```python
from build123d import *

# Parameters (mm, degrees)
SKETCH2_W            = 145.63575991
SKETCH2_H            = 16.06113598
BOSS_EXTRUDE1_DEPTH  = 80
SKETCH3_R            = 10
CUT_EXTRUDE1_DEPTH   = 110.363630747
BOSS_EXTRUDE2_DEPTH  = 20
SKETCH5_R            = 30
SKETCH5_R_2          = 10
BOSS_EXTRUDE3_DEPTH  = 100
FILLET1_R            = 5
BOSS_EXTRUDE9_REACH  = 183.085
BOSS_EXTRUDE10_DEPTH = 10
FILLET2_R            = 5
FILLET3_R            = 30


with BuildPart() as part:
    # Sketch2 → Boss-Extrude1 (new, symmetric)
    with BuildSketch(Plane(origin=(0, 0, 0), x_dir=(0, 0, -1), z_dir=(1, 0, 0))):
        Rectangle(SKETCH2_W, SKETCH2_H)
    extrude(amount=BOSS_EXTRUDE1_DEPTH, both=True)

    # Sketch3 → Cut-Extrude1 (cut, through all)
    with BuildSketch(Plane(origin=(0, 8.03056799, 0), x_dir=(1, 0, 0), z_dir=(0, 1, 0))):
        with Locations(Location((50, -42.817879955, 0), (0, 0, 270))):
            Circle(SKETCH3_R)
        with Locations(Location((-50, -42.817879955, 0), (0, 0, 270))):
            Circle(SKETCH3_R)
    extrude(amount=-CUT_EXTRUDE1_DEPTH, mode=Mode.SUBTRACT)

    # Sketch4 → Boss-Extrude2 (add)
    with BuildSketch(Plane(origin=(0, 0, -72.817879955), x_dir=(-1, 0, 0), z_dir=(0, 0, -1))):
        with BuildLine():
            Line((-26.680786367, 111.746822538), (-80, 8.03056799))
            Line((-80, 8.03056799), (80, 8.03056799))
            Line((80, 8.03056799), (26.680786367, 111.746822538))
            ThreePointArc((26.680786367, 111.746822538), (29.158391511, 105.086643705), (30, 98.03056799))
            ThreePointArc((30, 98.03056799), (-7.056075715, 68.872176479), (-26.680786367, 111.746822538))
        make_face()
    extrude(amount=-BOSS_EXTRUDE2_DEPTH)

    # Sketch5 → Boss-Extrude3 (add)
    with BuildSketch(Plane(origin=(0, 0, -72.817879955), x_dir=(-1, 0, 0), z_dir=(0, 0, -1))):
        with Locations((0, 98.03056799)):
            Circle(SKETCH5_R)
        with Locations((0, 98.03056799)):
            Circle(SKETCH5_R_2, mode=Mode.SUBTRACT)
    extrude(amount=-BOSS_EXTRUDE3_DEPTH)

    # Fillet1
    fillet1_edges = [part.edges().sort_by_distance(p)[0] for p in [
        (0, 8.03056799, -52.817879955),
    ]]
    fillet(fillet1_edges, radius=FILLET1_R)

    # Boss-Extrude9: up to this face of the body (flat: up to its plane)
    boss_extrude9_end = Plane(part.part.faces().sort_by_distance((0, 43.997298741, -52.817879955))[0])
    # Sketch12 → Boss-Extrude9 (add, up to the picked face)
    with BuildSketch(Plane.XY.offset(27.182120045), mode=Mode.PRIVATE) as boss_extrude9_sk1:
        with BuildLine():
            Line((10, 69.746296743), (10, 8.03056799))
            Line((10, 8.03056799), (-10, 8.03056799))
            Line((-10, 8.03056799), (-10, 69.746296743))
            ThreePointArc((-10, 69.746296743), (0, 68.03056799), (10, 69.746296743))
        make_face()
    boss_extrude9_tool1 = split(extrude(boss_extrude9_sk1.sketch, amount=-BOSS_EXTRUDE9_REACH, mode=Mode.PRIVATE), bisect_by=boss_extrude9_end, keep=Keep.BOTH, mode=Mode.PRIVATE)
    add(boss_extrude9_tool1.solids().sort_by(Axis((0, 38.315311, 27.18212), (0, 0, -1)))[0])

    # Sketch14 → Boss-Extrude10 (add, symmetric)
    with BuildSketch(Plane(origin=(0, 0, 0), x_dir=(0, 0, -1), z_dir=(1, 0, 0))):
        Polygon((-27.182120045, 69.746296743), (-72.817879955, 8.03056799), (-27.182120045, 8.03056799), align=None)
    extrude(amount=BOSS_EXTRUDE10_DEPTH, both=True)

    # Fillet2
    # the kernel refuses this fillet: 5 mm, written as the material it adds along each edge
    with BuildSketch(Plane(origin=(10, 13.03056799, -47.817879955), x_dir=(0, 0, -1), z_dir=(0, 1, 0))) as fillet2_piece_1:
        with BuildLine():
            CenterArc((5 - FILLET2_R, -FILLET2_R), FILLET2_R, 0, 90)
            Line((5, -FILLET2_R), (5, 0))
            Line((5, 0), (5 - FILLET2_R, 0))
        make_face()
    revolve(axis=Axis((10, 13.03056799, -47.817879955), (-1, 0, 0)), revolution_arc=90)
    with BuildSketch(Plane(origin=(-10, 13.03056799, -47.817879955), x_dir=(0, 0, -1), z_dir=(0, 1, 0))) as fillet2_piece_2:
        with BuildLine():
            CenterArc((5 - FILLET2_R, FILLET2_R), FILLET2_R, 270, 90)
            Line((5, FILLET2_R), (5, 0))
            Line((5, 0), (5 - FILLET2_R, 0))
        make_face()
    revolve(axis=Axis((-10, 13.03056799, -47.817879955), (-1, 0, 0)), revolution_arc=90)
    with BuildSketch(Plane(origin=(-10, 8.03056799, 72.817879955), x_dir=(-1, 0, 0), z_dir=(0, 0, -1))) as fillet2_piece_3_section:
        with BuildLine():
            CenterArc((FILLET2_R, FILLET2_R), FILLET2_R, 180, 90)
            Line((0, FILLET2_R), (0, 0))
            Line((0, 0), (FILLET2_R, 0))
        make_face()
    fillet2_piece_3 = extrude(amount=120.63575991, mode=Mode.PRIVATE)
    fillet2_piece_3 = split(fillet2_piece_3, bisect_by=Plane(origin=(-10, 8.03056799, 72.817879955), z_dir=(0, -0.5945577575874679, -0.8040529042871258)), keep=Keep.TOP, mode=Mode.PRIVATE)
    add(fillet2_piece_3)
    with BuildSketch(Plane(origin=(-10, 82.246296743, -52.817879955), x_dir=(0, 0, 1), z_dir=(0, -1, 0))) as fillet2_piece_4:
        with BuildLine():
            CenterArc((FILLET2_R, FILLET2_R), FILLET2_R, 180, 90)
            Line((0, FILLET2_R), (0, 0))
            Line((0, 0), (FILLET2_R, 0))
        make_face()
    extrude(amount=69.215728753)
    with BuildSketch(Plane(origin=(10, 13.03056799, -52.817879955), x_dir=(1, 0, 0), z_dir=(0, 1, 0))) as fillet2_piece_5:
        with BuildLine():
            CenterArc((FILLET2_R, -FILLET2_R), FILLET2_R, 90, 90)
            Line((0, -FILLET2_R), (0, 0))
            Line((0, 0), (FILLET2_R, 0))
        make_face()
    extrude(amount=69.215728753)
    with BuildSketch(Plane(origin=(10, 8.03056799, -47.817879955), x_dir=(1, 0, 0), z_dir=(0, 0, 1))) as fillet2_piece_6_section:
        with BuildLine():
            CenterArc((FILLET2_R, FILLET2_R), FILLET2_R, 180, 90)
            Line((0, FILLET2_R), (0, 0))
            Line((0, 0), (FILLET2_R, 0))
        make_face()
    fillet2_piece_6 = extrude(amount=120.63575991, mode=Mode.PRIVATE)
    fillet2_piece_6 = split(fillet2_piece_6, bisect_by=Plane(origin=(10, 65.701203771, 30.173268256), z_dir=(0, -0.5945577575874679, -0.8040529042871258)), keep=Keep.TOP, mode=Mode.PRIVATE)
    add(fillet2_piece_6)

    # Fillet3
    fillet3_edges = [part.edges().sort_by_distance(p)[0] for p in [
        (80, 0, 72.817879955),
        (-80, 0, 72.817879955),
    ]]
    fillet(fillet3_edges, radius=FILLET3_R)


solid = part.part
```
Source: CAD feature listing. Evaluate the final solid. Frame: model axes, mm. A direction names the side the tool comes from. Coordinates: 2 decimals unless noted, no trailing zeros. Loops run counter-clockwise (first coordinate to the right, second up) from the corner with the lowest first, then second, coordinate; pieces in that order, holes last. Notation, with made-up numbers: M 70,33 L 98,33 A25 cw 98,63 Z; hole C 54,63 d11. An arc over 180 degrees is marked long. Put each result on its own line as item: value. Start each with the question number.
1) Cut plane B-B on z = -19. Return the cut outline in (x, y).
2) Contact query for flat-ended pins moving along their axis: pin 1 Ø19.5 at (x, z) = (57, 5.5) entering from +Y; pin 2 Ø1.5 at (y, z) = (70, -38.5) entering from -X; pin 3 Ø5 at (y, z) = (14, -57) entering from -X. Output: stop coordinate, or through.
3) Cut plane A-A on x = 0. Return the cut outline in (y, z), then the cut area to 3 significant figures.
4) Reachability of faces 4 (the face through (-80, 0, -14)), 5 (the face through (-39, 41, -52.818)), 6 (the face through (10, 42, -2)) from +Z, -Z, +X, -X, +Y, -Y: full face, straight path, thin tool, end or side. Return the list, or none.
5) Cut plane D-D on y = 34.5. Return the cut outline in (x, z), then the cut area to 3 significant figures.
6) Ray query, L1, parallel to Y at x = 0, z = -26.5; L2, parallel to X at y = 33.5, z = -28.5; L3, parallel to Y at x = -54, z = -45. Return the intervals inside material, ascending. Write a range as from..to.
7) Pull-direction query (X, two-part tool) for faces 1 (the face through (11.43, 9.53, 11.66)), 2 (the face through (-11.5, 42.95, -51.39)), 3 (the face through (-4.614, 89.159, -23.518)); classes: pulls with the +X half, pulls with the -X half, needs draft (parallel to the pull), parting line crosses it, or undercut.
8) Cut plane C-C on z = 35.5. Return the cut outline in (x, y), then the cut area to 3 significant figures.
The answers:
1. outline: M -80,-8.03 L 80,-8.03 L 80,8.03 L 15,8.03 A5 cw 10,13.03 L 10,69.75 A30 ccw long -10,69.75 L -10,13.03 A5 cw -15,8.03 L -80,8.03 Z; hole C 0,98.03 d20
2. pin 1: stops at y = 8.03
2. pin 2: stops at x = -12.48
2. pin 3: stops at x = -78.22
3. outline: M -8.03,-72.82 L 88.03,-72.82 L 88.03,27.18 L 69.75,27.18 L 8.03,72.82 L -8.03,72.82 Z; M 108.03,-72.82 L 128.03,-72.82 L 128.03,27.18 L 108.03,27.18 Z
3. area: 13,700 mm²
4. face 4: +Z, -Z, -X, +Y, -Y
4. face 5: +Z, -X
4. face 6: +Z, +X
5. outline: M -66.39,-72.82 L 66.39,-72.82 L 66.39,-52.82 L 15,-52.82 A5 cw 10,-47.82 L 10,53.25 L -10,53.25 L -10,-47.82 A5 cw -15,-52.82 L -66.39,-52.82 Z
5. area: 4,790 mm²
6. L1: y = -8.03..88.03, 108.03..128.03
6. L2: x = -10..10
6. L3: y = -8.03..8.03
7. face 1: pulls with the +X half
7. face 2: pulls with the -X half
7. face 3: undercut
8. outline: M -80,-8.03 L -56.82,-8.03 L -56.82,8.03 L -80,8.03 Z; M -43.18,-8.03 L 43.18,-8.03 L 43.18,8.03 L 15,8.03 A5 cw 10,13.03 L 10,58.5 L -10,58.5 L -10,13.03 A5 cw -15,8.03 L -43.18,8.03 Z; M 56.82,-8.03 L 80,-8.03 L 80,8.03 L 56.82,8.03 Z
8. area: 3,150 mm²
